Check sheet for the drawn part. Datum: minimum x, y, z corner. Units: mm. A direction names the side the tool comes from. Round coordinates to 2 decimals unless told otherwise and drop trailing zeros. Write each loop counter-clockwise with the first axis right and the second up, starting at its lowest first coordinate (ties: lowest second). Pieces come first, ordered by that corner, then holes. Notation, with made-up numbers: (-9, 61) -> (2, 61) arc R23 cw to (2, 76) -> close; hole circle Ø7 at (-30, 40). An arc over 180 degrees is marked (long way). Use a Markdown table: item, result.
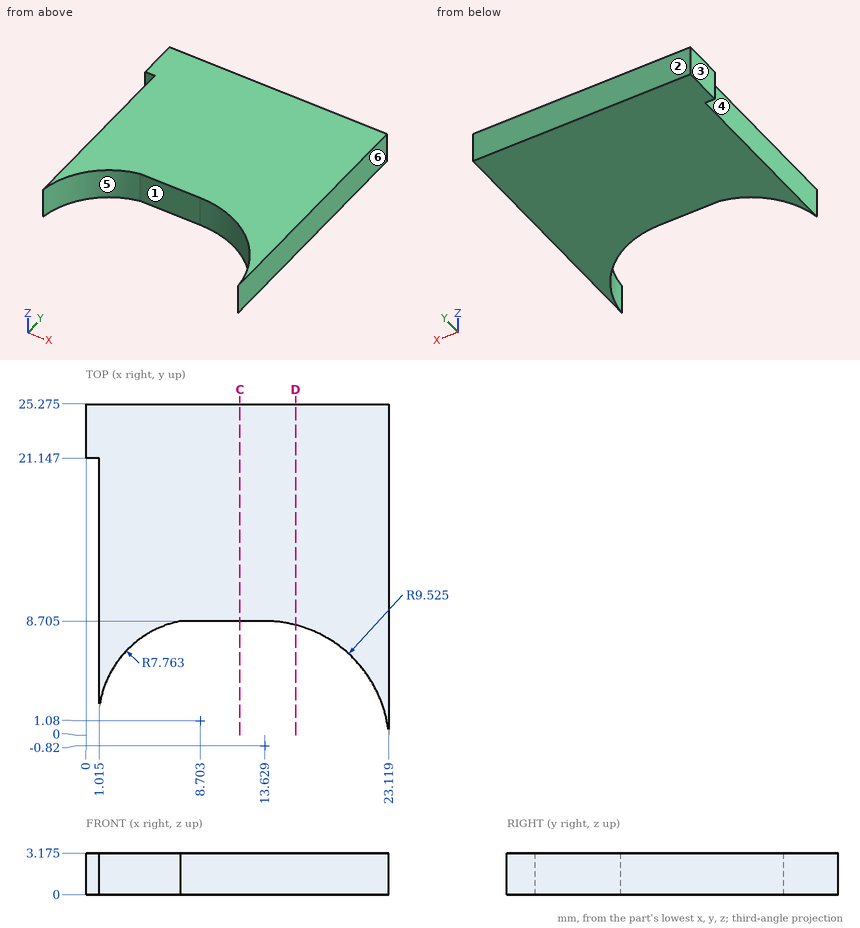
(1) Gauge pin test, flat ends, axial feed: pin 1 Ø1.6 at (y, z) = (14.5, 1.5) entering from -X (3 decimals); pin 2 Ø0.5 at (x, z) = (0.5, 1) entering from -Y; pin 3 Ø1.6 at (x, z) = (11, 2) entering from -Y (1 decimal). Record the tip position at first contact, or that the pin passes through.
A:
| item | result |
|---|---|
| pin 1 | stops at x = 1.015 |
| pin 2 | stops at y = 21.15 |
| pin 3 | stops at y = 8.7 |
(2) Access from +Z, -Z, +X, -X, +Y, -Y to the whole of each face (thin tool, end or side, straight path). Record for the marked faces 4, 5 and 6.
A:
| item | result |
|---|---|
| face 4 | +Z, -Z, -X, -Y |
| face 5 | +Z, -Z, -Y |
| face 6 | +Z, -Z, +X, +Y, -Y |
(3) Thickness scan on line 1 (Y direction, x = 9.25, z = 1.55) (1 decimal); line 2 (X direction, y = 14.5, z = 2.2) (1 decimal); line 3 (X direction, y = 5.25, z = 0.55) (1 decimal). Record the ranges inside material, lowest first.
A:
| item | result |
|---|---|
| line 1 | y = 8.7 to 25.3 |
| line 2 | x = 1 to 23.1 |
| line 3 | x = 1 to 2.2, 21 to 23.1 |
(4) Section check D-D on x = 16. Record the cut outline in (y, z) (1 decimal).
A:
| item | result |
|---|---|
| outline | (8.4, 0) -> (25.3, 0) -> (25.3, 3.2) -> (8.4, 3.2) -> close |
(5) Section check C-C on x = 11.75. Record the cut outline in (y, z) (1 decimal).
A:
| item | result |
|---|---|
| outline | (8.7, 0) -> (25.3, 0) -> (25.3, 3.2) -> (8.7, 3.2) -> close |
(6) Release check for a two-part mould opening along X. For the marked faces 1, 2 and 3 record: +X half, -X half, draft (parallel to the pull), parting line (faces both ways), or undercut.
A:
| item | result |
|---|---|
| face 1 | undercut |
| face 2 | draft |
| face 3 | -X half |
